Input: dimensioned drawing with shaded views. Units: mm. Origin: part minimum x, y, z. A direction names the side the tool comes from. Coordinates: 2 decimals unless noted, no trailing zeros. Write each loop counter-clockwise with the first axis right and the second up, starting at its lowest first coordinate (ties: lowest second). Pieces come first, ordered by that corner, then holes. Notation, with made-up numbers: M 73,7 L 118,7 A12 cw 118,13 Z; hole C 19.25,19.25 d10. An arc over 180 degrees is marked long. Write each question's results on one line, items separated by ' | '. Start each with the question number.
1. Section query C-C, the plane y = 2.35. Output: boundary loops of the cut face in (x, z).
2. Section query A-A, the plane x = 7.5. Output: boundary loops of the cut face in (y, z).
3. Section query D-D, the plane y = 4.6. Output: boundary loops of the cut face in (x, z) (1 decimal), and give its area (3 significant figures).
4. Pull-direction query (X, two-part tool) for the marked faces 1, 2, 3 and 4; classes: +X half, -X half, draft (parallel to the pull), parting line (faces both ways), or undercut.
5. Section query B-B, the plane z = 1.4. Output: boundary loops of the cut face in (x, y) (1 decimal).
6. Ray query, probe 1 along X at (y, z) = (2.65, 0.25); probe 2 along Y at (x, z) = (7.5, 1.25); probe 3 along Y at (x, z) = (12.25, 1.15). Return the intervals inside material, ascending.
7. Set-up query: the marked faces 5 and 6. Return all of +Z, -Z, +X, -X, +Y, -Y with unobstructed straight access to the full face (end or side cutting, diameter ignored); none if empty.
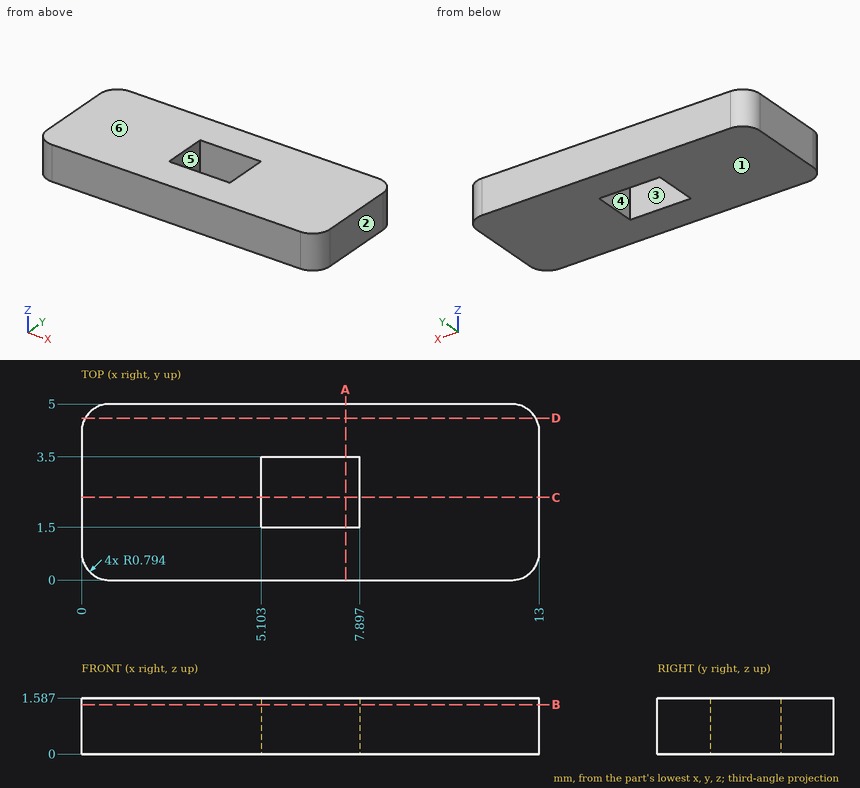
Answer:
1) outline: M 0,0 L 5.1,0 L 5.1,1.59 L 0,1.59 Z; M 7.9,0 L 13,0 L 13,1.59 L 7.9,1.59 Z
2) outline: M 0,0 L 1.5,0 L 1.5,1.59 L 0,1.59 Z; M 3.5,0 L 5,0 L 5,1.59 L 3.5,1.59 Z
3) outline: M 0.1,0 L 12.9,0 L 12.9,1.6 L 0.1,1.6 Z | area: 20.3 mm^2
4) face 1: draft | face 2: +X half | face 3: undercut | face 4: undercut
5) outline: M 0,0.8 A0.8 ccw 0.8,0 L 12.2,0 A0.8 ccw 13,0.8 L 13,4.2 A0.8 ccw 12.2,5 L 0.8,5 A0.8 ccw 0,4.2 Z; hole M 5.1,1.5 L 7.9,1.5 L 7.9,3.5 L 5.1,3.5 Z
6) probe 1: 0 to 5.1, 7.9 to 13 | probe 2: 0 to 1.5, 3.5 to 5 | probe 3: 0 to 5
7) face 5: +Z, -Z | face 6: +Z, +X, -X, +Y, -Y
